Here's how the part is built. I have some questions about the finished solid (model axes, mm). Face numbers are marked on the shaded views. A direction names the side the tool comes from. Coordinates: 2 decimals unless noted, no trailing zeros. Write each loop counter-clockwise with the first axis right and the second up, starting at its lowest first coordinate (ties: lowest second). Pieces come first, ordered by that corner, then holes.
Item 1: For the marked faces 4, 5 and 6, which set-ups out of +Z, -Z, +X, -X, +Y, -Y let a thin tool reach every point of the face, with its end or its side?
Item 2: If we mould it in two halves opening along Y, with no side actions, what happens to the marked faces 1, 2 and 3? For each: pulls with the +Y half, pulls with the -Y half, needs draft (parallel to the pull), parting line crosses it, or undercut.
Item 3: Please list where these lines run through material, in increasing order: line 1 (X direction, y = 4.25, z = 25); line 2 (Z direction, x = 55, y = 0.5); line 3 (X direction, y = 4.75, z = 24).
Item 4: I want a section at D-D (x = 9.5). Please give me the cut outline in (y, z).
Item 5: I'm going to push flat-ended pins straight in: P1, Ø21, axis at x = 60, z = -25, coming from the +Y side; P2, Ø2.5, axis at y = 12, z = -16.5, coming from the +X side; P3, Ø1.5, axis at y = 12, z = 17, coming from the -X side. Where does each tip first touch, or does it pass through?
Item 6: I want a section at B-B (z = -28). Please give me the cut outline in (x, y).
Item 7: I want a section at A-A (y = 5). Please give me the cut outline in (x, z), and give its area (3 significant figures).
Item 8: I want a section at C-C (z = 16.5). Please give me the cut outline in (x, y).
from build123d import *

# Parameters (mm, degrees)
CROQUIS2_W              = 146
CROQUIS2_H              = 76
SALIENTE_EXTRUIR2_DEPTH = 10
CROQUIS3_W              = 66
CROQUIS3_H              = 76
SALIENTE_EXTRUIR3_DEPTH = 3
REDONDEO1_R             = 13
REDONDEO2_R             = 13
REDONDEO3_R             = 13
REDONDEO4_R             = 13
CROQUIS5_R              = 6.5
CORTAR_EXTRUIR1_DEPTH   = 83.903558428
CROQUIS6_W              = 72
CROQUIS6_H              = 76
CORTAR_EXTRUIR2_DEPTH   = 3
CHAFL_N1_SIZE           = 4
CHAFL_N2_SIZE           = 4


with BuildPart() as part:
    # Croquis2 → Saliente-Extruir2 (new body)
    with BuildSketch(Plane(origin=(0, 0, 0), x_dir=(1, 0, 0), z_dir=(0, 1, 0))):
        Rectangle(CROQUIS2_W, CROQUIS2_H)
    extrude(amount=SALIENTE_EXTRUIR2_DEPTH)

    # Croquis3 → Saliente-Extruir3 (add)
    with BuildSketch(Plane(origin=(0, 10, 0), x_dir=(1, 0, 0), z_dir=(0, 1, 0))):
        Rectangle(CROQUIS3_W, CROQUIS3_H)
    extrude(amount=SALIENTE_EXTRUIR3_DEPTH)

    # Redondeo1
    redondeo1_edges = [part.edges().sort_by_distance(p)[0] for p in [
        (-73, 5, -38),
    ]]
    fillet(redondeo1_edges, radius=REDONDEO1_R)

    # Redondeo2
    redondeo2_edges = [part.edges().sort_by_distance(p)[0] for p in [
        (-73, 5, 38),
    ]]
    fillet(redondeo2_edges, radius=REDONDEO2_R)

    # Redondeo3
    redondeo3_edges = [part.edges().sort_by_distance(p)[0] for p in [
        (73, 5, 38),
    ]]
    fillet(redondeo3_edges, radius=REDONDEO3_R)

    # Redondeo4
    redondeo4_edges = [part.edges().sort_by_distance(p)[0] for p in [
        (73, 5, -38),
    ]]
    fillet(redondeo4_edges, radius=REDONDEO4_R)

    # Croquis5 → Cortar-Extruir1 (cut, through all)
    with BuildSketch(Plane(origin=(0, 10, 0), x_dir=(1, 0, 0), z_dir=(0, 1, 0))):
        with Locations(Location((-60, 25, 0), (0, 0, 270))):
            Circle(CROQUIS5_R)
        with Locations(Location((-60, -25, 0), (0, 0, 270))):
            Circle(CROQUIS5_R)
        with Locations(Location((60, -25, 0), (0, 0, 270))):
            Circle(CROQUIS5_R)
        with Locations(Location((60, 25, 0), (0, 0, 270))):
            Circle(CROQUIS5_R)
    extrude(amount=-CORTAR_EXTRUIR1_DEPTH, mode=Mode.SUBTRACT)

    # Croquis6 → Cortar-Extruir2 (cut)
    with BuildSketch(Plane.XZ):
        Rectangle(CROQUIS6_W, CROQUIS6_H)
    extrude(amount=-CORTAR_EXTRUIR2_DEPTH, mode=Mode.SUBTRACT)

    # Chaflán1
    # the kernel refuses this chamfer: 4 mm, written as the material it adds along each edge
    with BuildSketch(Plane(origin=(-36, 3, 38), x_dir=(-0.027495876610585623, -0.9996219169112968, 0), z_dir=(0, 0, -1))) as chafl_n1_piece_1_section:
        Polygon((CHAFL_N1_SIZE * 0.999621916911, -CHAFL_N1_SIZE * 0.0274958766106), (-CHAFL_N1_SIZE * 0.0274958766106, -CHAFL_N1_SIZE * 0.999621916911), (0, 0), align=None)
    chafl_n1_piece_1 = extrude(amount=76, mode=Mode.PRIVATE)
    chafl_n1_piece_1 = split(chafl_n1_piece_1, bisect_by=Plane(origin=(-34.592163559, 0, 0), z_dir=(0, 1, 0)), keep=Keep.TOP, mode=Mode.PRIVATE)
    add(chafl_n1_piece_1)

    # Chaflán2
    # the kernel refuses this chamfer: 4 mm, written as the material it adds along each edge
    with BuildSketch(Plane(origin=(36, 3, -38), x_dir=(0.027495876610585623, -0.9996219169112968, 0), z_dir=(0, 0, 1))) as chafl_n2_piece_1_section:
        Polygon((CHAFL_N2_SIZE * 0.999621916911, -CHAFL_N2_SIZE * 0.0274958766106), (-CHAFL_N2_SIZE * 0.0274958766106, -CHAFL_N2_SIZE * 0.999621916911), (0, 0), align=None)
    chafl_n2_piece_1 = extrude(amount=76, mode=Mode.PRIVATE)
    chafl_n2_piece_1 = split(chafl_n2_piece_1, bisect_by=Plane(origin=(34.592163559, 0, 0), z_dir=(0, 1, 0)), keep=Keep.TOP, mode=Mode.PRIVATE)
    add(chafl_n2_piece_1)


solid = part.part
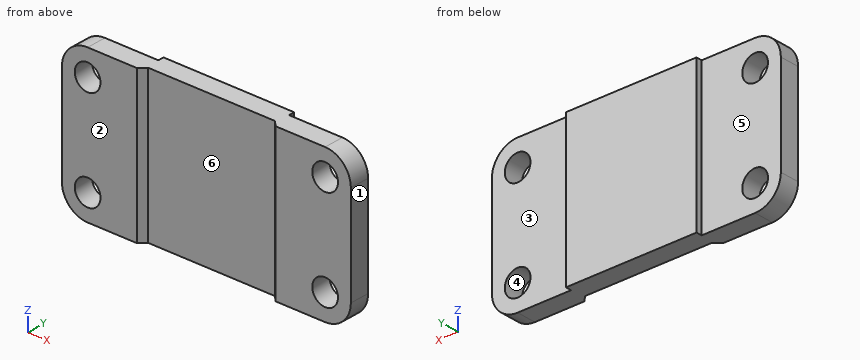
Answer:
1. face 4: +Y, -Y
1. face 5: +Z, -Z, -X, +Y
1. face 6: +Z, -Z, -Y
2. face 1: needs draft
2. face 2: pulls with the -Y half
2. face 3: pulls with the +Y half
3. line 1: x = -73 to -66.5, -53.5 to 53.5, 66.5 to 73
3. line 2: z = -38 to -29.15, -20.85 to 20.85, 29.15 to 38
3. line 3: x = -73 to -66.42, -53.58 to 53.58, 66.42 to 73
4. outline: (3, -38) - (13, -38) - (13, 38) - (3, 38) - close
5. P1: stops at y = 10
5. P2: stops at x = 33
5. P3: stops at x = -33
6. outline: (-72.65, 0) - (-65.77, 0) - (-65.77, 10) - (-72.65, 10) - close; (-54.23, 0) - (-35, 0) - (-32, 3) - (32, 3) - (35, 0) - (54.23, 0) - (54.23, 10) - (33, 10) - (33, 13) - (-33, 13) - (-33, 10) - (-54.23, 10) - close; (65.77, 0) - (72.65, 0) - (72.65, 10) - (65.77, 10) - close
7. outline: (-73, -25) arc R13 ccw to (-60, -38) - (60, -38) arc R13 ccw to (73, -25) - (73, 25) arc R13 ccw to (60, 38) - (-60, 38) arc R13 ccw to (-73, 25) - close; hole circle Ø13 at (-60, -25); hole circle Ø13 at (-60, 25); hole circle Ø13 at (60, -25); hole circle Ø13 at (60, 25)
7. area: 10,400 mm2
8. outline: (-73, 0) - (-35, 0) - (-32, 3) - (32, 3) - (35, 0) - (73, 0) - (73, 10) - (33, 10) - (33, 13) - (-33, 13) - (-33, 10) - (-73, 10) - close
